from build123d import *

# Parameters (mm, degrees)
F1_DEPTH = 304.8


with BuildPart() as f1:
    # F0 (on Front) → F1 (new body)
    with BuildSketch(Plane.XZ):
        with BuildLine():
            Line((-5.08, 0), (0, 0))
            Line((0, 0), (5.08, 0))
            Line((5.08, 0), (5.08, 1.905))
            Line((5.08, 1.905), (1.016, 3.175))
            Line((1.016, 3.175), (1.016, 8.89))
            Line((1.016, 8.89), (3.81, 10.16))
            Line((3.81, 10.16), (3.81, 11.43))
            ThreePointArc((3.81, 11.43), (3.574513, 12.080427), (2.977213, 12.429344))
            ThreePointArc((2.977213, 12.429344), (1.494745, 12.632197), (0, 12.7))
            ThreePointArc((0, 12.7), (-1.494745, 12.632197), (-2.977213, 12.429344))
            ThreePointArc((-2.977213, 12.429344), (-3.574513, 12.080427), (-3.81, 11.43))
            Line((-3.81, 11.43), (-3.81, 10.16))
            Line((-3.81, 10.16), (-1.016, 8.89))
            Line((-1.016, 8.89), (-1.016, 3.175))
            Line((-1.016, 3.175), (-5.08, 1.905))
            Line((-5.08, 1.905), (-5.08, 0))
        make_face()
    extrude(amount=F1_DEPTH)


solid = f1.part
Geometry: final body of the model. Coordinates: model frame, mm. Coordinates: 2 decimals unless noted, no trailing zeros. Write each loop counter-clockwise with the first axis right and the second up, starting at its lowest first coordinate (ties: lowest second). Pieces come first, ordered by that corner, then holes. Notation, with made-up numbers: (-1, 15.5) - (26, 15.5) arc R8 ccw to (26, 21.5) - close; hole circle Ø8 at (50.5, 59.25). An arc over 180 degrees is marked (long way). Return JSON: item names as keys, results as strings.
Item 1: Section query A-A (y = -271.5). Output: boundary loops of the cut face in (x, z) (3 decimals).
Completed:
{"outline": "(-5.08, 0) - (5.08, 0) - (5.08, 1.905) - (1.016, 3.175) - (1.016, 8.89) - (3.81, 10.16) - (3.81, 11.43) arc R1.016 ccw to (2.977, 12.429) arc R16.51 ccw to (0, 12.7) arc R16.51 ccw to (-2.977, 12.429) arc R1.016 ccw to (-3.81, 11.43) - (-3.81, 10.16) - (-1.016, 8.89) - (-1.016, 3.175) - (-5.08, 1.905) - close"}
Item 2: Pull-direction query (X, two-part tool) for faces 1 (the face through (0, -304.8, 6)), 2 (the face through (1.016, -150, 6)), 3 (the face through (-1.016, -150, 6)); classes: +X half, -X half, draft (parallel to the pull), parting line (faces both ways), or undercut.
Completed:
{"face 1": "draft", "face 2": "+X half", "face 3": "-X half"}
Item 3: Line query: L1, parallel to X at y = -287, z = 11; L2, parallel to X at y = -33, z = 8.75; L3, parallel to Z at x = -2.5, y = -271. Output: solid intervals per line, ascending.
Completed:
{"L1": "x = -3.81 to 3.81", "L2": "x = -1.02 to 1.02", "L3": "z = 0 to 2.71, 9.56 to 12.51"}
Item 4: Pin query (flat end, axial travel): pin 1 Ø1 at (x, z) = (3, 9) entering from +Y; pin 2 Ø4 at (y, z) = (-233, 10) entering from +X; pin 3 Ø0.6 at (y, z) = (-200, 11) entering from -X. Return the tip coordinate at first contact, or that it passes through.
Completed:
{"pin 1": "passes through", "pin 2": "stops at x = 3.81", "pin 3": "stops at x = -3.81"}
